from build123d import *

# Parameters (mm, degrees)
F1_DEPTH = 25.4


with BuildPart() as f1:
    # F0 (on Front) → F1 (new body)
    with BuildSketch(Plane.XZ):
        with BuildLine():
            Line((72.0466873491, 0), (40.2231729678, -21.8466586519))
            ThreePointArc((40.2231729678, -21.8466586519), (31.3848696272, -33.3192151219), (19.4048266012, -41.4563968819))
            ThreePointArc((19.4048266012, -41.4563968819), (33.8870469148, -41.4351204215), (47.6510526714, -45.9392633402))
            Line((47.6510526714, -45.9392633402), (86.2514989391, -46.0738358679))
            Line((86.2514989391, -46.0738358679), (115.6003371528, -26.0762075411))
            ThreePointArc((115.6003371528, -26.0762075411), (109.6163777827, -13.6436900901), (107.560902013, 0))
            Line((107.560902013, 0), (72.0466873491, 0))
        make_face()
        with BuildLine():
            Line((127.6607268874, 38.1787166397), (72.0466873491, 0))
            Line((72.0466873491, 0), (107.560902013, 0))
            ThreePointArc((107.560902013, 0), (112.8928076077, 21.5732320494), (127.6607268874, 38.1787166397))
        make_face()
        with BuildLine():
            ThreePointArc((47.6510526714, -45.9392633402), (33.8870469148, -41.4351204215), (19.4048266012, -41.4563968819))
            ThreePointArc((19.4048266012, -41.4563968819), (13.4857274503, -43.7414596577), (7.3075106005, -45.1860645185))
            ThreePointArc((7.3075106005, -45.1860645185), (6.6804139573, -45.4854183946), (6.0579339451, -45.7942574747))
            Line((6.0579339451, -45.7942574747), (47.6510526714, -45.9392633402))
        make_face()
        with BuildLine():
            ThreePointArc((64.5391180148, -60.8681565374), (57.0284030969, -52.3479095519), (47.6510526714, -45.9392633402))
            Line((47.6510526714, -45.9392633402), (6.0579339451, -45.7942574747))
            ThreePointArc((6.0579339451, -45.7942574747), (3.4488790791, -47.2217605692), (0.9380323387, -48.8156805874))
            ThreePointArc((0.9380323387, -48.8156805874), (-11.1144436113, -112.4167662635), (52.4866420648, -124.4692422135))
            ThreePointArc((52.4866420648, -124.4692422135), (67.1780692741, -108.036494814), (72.4854749339, -86.6424614004))
            ThreePointArc((72.4854749339, -86.6424614004), (70.4537968594, -73.1567339501), (64.5391180148, -60.8681565374))
        make_face()
        with BuildLine():
            Line((153.8701951504, 0), (107.560902013, 0))
            ThreePointArc((107.560902013, 0), (109.6163777827, -13.6436900901), (115.6003371528, -26.0762075411))
            Line((115.6003371528, -26.0762075411), (153.8701951504, 0))
        make_face()
        with BuildLine():
            ThreePointArc((40.2231729678, -21.8466586519), (44.3639548177, -11.2702994984), (45.7731377322, 0))
            ThreePointArc((45.7731377322, 0), (32.3664960866, 32.3664960866), (0, 45.7731377322))
            ThreePointArc((0, 45.7731377322), (-45.7731377322, 0), (0, -45.7731377322))
            ThreePointArc((0, -45.7731377322), (2.9724733003, -45.676520668), (5.932398121, -45.3870773501))
            Line((5.932398121, -45.3870773501), (40.2231729678, -21.8466586519))
        make_face()
        with BuildLine():
            ThreePointArc((0, 45.7731377322), (32.3664960866, 32.3664960866), (45.7731377322, 0))
            Line((45.7731377322, 0), (72.0466873491, 0))
            Line((72.0466873491, 0), (127.6607268874, 38.1787166397))
            ThreePointArc((127.6607268874, 38.1787166397), (140.0723070667, 44.2059828), (153.7087482925, 46.3090117126))
            Line((153.7087482925, 46.3090117126), (0, 45.7731377322))
        make_face()
        with BuildLine():
            ThreePointArc((19.4048266012, -41.4563968819), (31.3848696272, -33.3192151219), (40.2231729678, -21.8466586519))
            Line((40.2231729678, -21.8466586519), (5.932398121, -45.3870773501))
            ThreePointArc((5.932398121, -45.3870773501), (6.6207172783, -45.2917899908), (7.3075106005, -45.1860645185))
            ThreePointArc((7.3075106005, -45.1860645185), (13.2266097514, -42.9010017427), (19.4048266012, -41.4563968819))
        make_face()
        with BuildLine():
            ThreePointArc((7.3075106005, -45.1860645185), (13.4857274503, -43.7414596577), (19.4048266012, -41.4563968819))
            ThreePointArc((19.4048266012, -41.4563968819), (13.2266097514, -42.9010017427), (7.3075106005, -45.1860645185))
        make_face()
    extrude(amount=F1_DEPTH)


solid = f1.part
Design review of the part built by this model. Coordinates are the model's own, in mm. A direction names the side the tool comes from. Give positions to 0.01 mm unless a question says otherwise; leave off trailing zeros. Loops run counter-clockwise (first coordinate to the right, second up) from the corner with the lowest first, then second, coordinate; pieces in that order, holes last. Notation, with made-up numbers: (68.25, -31) - (117.25, -31) arc R18 cw to (117.25, -8) - close; hole circle Ø1 at (69, -38). An arc over 180 degrees is marked (long way). Use CSV: the item, a comma, the result in double quotes. Start each with the question number.
1. Insertion check: P1, Ø10, axis at x = 73.5, y = -5.5, coming from the +Z side; P2, Ø1.5, axis at x = 46, y = -16.5, coming from the +Z side; P3, Ø8, axis at x = -25, y = -15.5, coming from the +Z side. Each pin has a flat end and moves straight along its axis. Give the tip position at first contact, or say it passes through.
2. Wall thickness on L1, parallel to Z at x = 63, y = -7; L2, parallel to Z at x = 65, y = -11.75; L3, parallel to Z at x = 6.5, y = -16.25: over which ranges is each line inside the solid? List them lowest first.
3. Add section C-C (y = -21.5). State the section outline as (x, z) points, plus the area to 3 significant figures.
4. Draft analysis for pull direction Z (two halves, no side actions). For faces 1 (the flat face through (59, -13, 0)), 2 (the flat face through (30, 0, -22)), state which applies: released by +Z, released by -Z, zero draft, split by the parting line, or undercut.
5. Add section B-B (x = 137). State the section outline as (y, z) points.
6. Machinability: for faces 3 (the flat face through (56.36, -12.52, -10.77)), 4 (the flat face through (131, -13, 0)), 5 (the flat face through (30, -25.4, -22)), which of the approach directions +Z, -Z, +X, -X, +Y, -Y give a long, thin tool a straight path to every point of the face, cutting with its end or side? Answer none if there is none.
7. Add section A-A (z = -10). State the section outline as (x, y) points.
8. Add section D-D (z = 35). State the section outline as (x, y) points, plus the area to 3 significant figures.
Results found:
1,P1,"stops at z = 46.05"
1,P2,"stops at z = 45.94"
1,P3,"stops at z = 40.67"
2,L1,"z = -114.54 to -58.74, -45.99 to -6.21, 0 to 45.99"
2,L2,"z = -111.73 to -61.56, -46 to -4.84, 0 to 46"
2,L3,"z = -127.71 to -45.57, -45.31 to 45.8"
3,outline,"(0, 45.77) arc R45.77 ccw (long way) to (7.31, -45.19) arc R45.77 ccw (long way) to (47.65, -45.94) - (86.25, -46.07) - (153.87, 0) - (107.56, 0) arc R46.31 cw to (153.71, 46.31) - close; hole (40.22, -21.85) - (72.05, 0) - (45.77, 0) arc R45.77 cw to start"
3,area,"20,400 mm²"
4,face 1,"undercut"
4,face 2,"zero draft"
5,outline,"(-25.4, -11.49) - (0, -11.49) - (0, 0) - (-25.4, 0) - close; (-25.4, 43.13) - (0, 43.13) - (0, 46.25) - (-25.4, 46.25) - close"
6,face 3,"+Y, -Y"
6,face 4,"+X, +Y, -Y"
6,face 5,"+Z, -Z, +X, -X, -Y"
7,outline,"(-44.67, -25.4) - (44.67, -25.4) - (44.67, 0) - (-44.67, 0) - close; (57.48, -25.4) - (139.19, -25.4) - (139.19, 0) - (57.48, 0) - close"
8,outline,"(-29.5, -25.4) - (123.55, -25.4) - (123.55, 0) - (-29.5, 0) - close"
8,area,"3,890 mm²"
